The figure shows three views and two pictorial views of one solid part (mm, origin at its lowest corner). Answer the questions. A direction names the side the tool comes from. Give positions to 0.01 mm unless a question says otherwise; leave off trailing zeros. Write each loop counter-clockwise with the first axis right and the second up, starting at its lowest first coordinate (ties: lowest second). Pieces come first, ordered by that corner, then holes. Notation, with made-up numbers: (83.5, 18) - (110.5, 18) arc R23 ccw to (110.5, 35) - close; hole circle Ø4 at (43, 8). An arc over 180 degrees is marked (long way). One line per question, with ' | ' between items. Start each with the question number.
1. A cutting plane is placed at C-C (x = 1.5). Determine the outline of the cut face in (y, z).
2. Given P1, Ø1, axis at x = 1.5, z = 5.5, coming from the -Y side; P2, Ø1, axis at x = 10.5, z = 7, coming from the -Y side; P3, Ø5, axis at x = 11.5, z = 4, coming from the -Y side, each flat-ended and moving along its own axis, determine where each tip first touches the part or whether it passes through.
3. A cutting plane is placed at D-D (x = 10). Determine the outline of the cut face in (y, z), then the cut area to 3 significant figures.
4. Find the intervals of material crossed by L1, parallel to Z at x = 2.25, y = 4.75; L2, parallel to Z at x = 6.75, y = 6.75; L3, parallel to Y at x = 7.75, z = 3, in increasing order. Write a range as from..to.
5. A cutting plane is placed at A-A (y = 4.7). Determine the outline of the cut face in (x, z), then the cut area to 3 significant figures.
6. For the marked faces 1 and 2, determine the directions among +Z, -Z, +X, -X, +Y, -Y from which every point of the face is accessible in a straight line to the end or side of a thin tool.
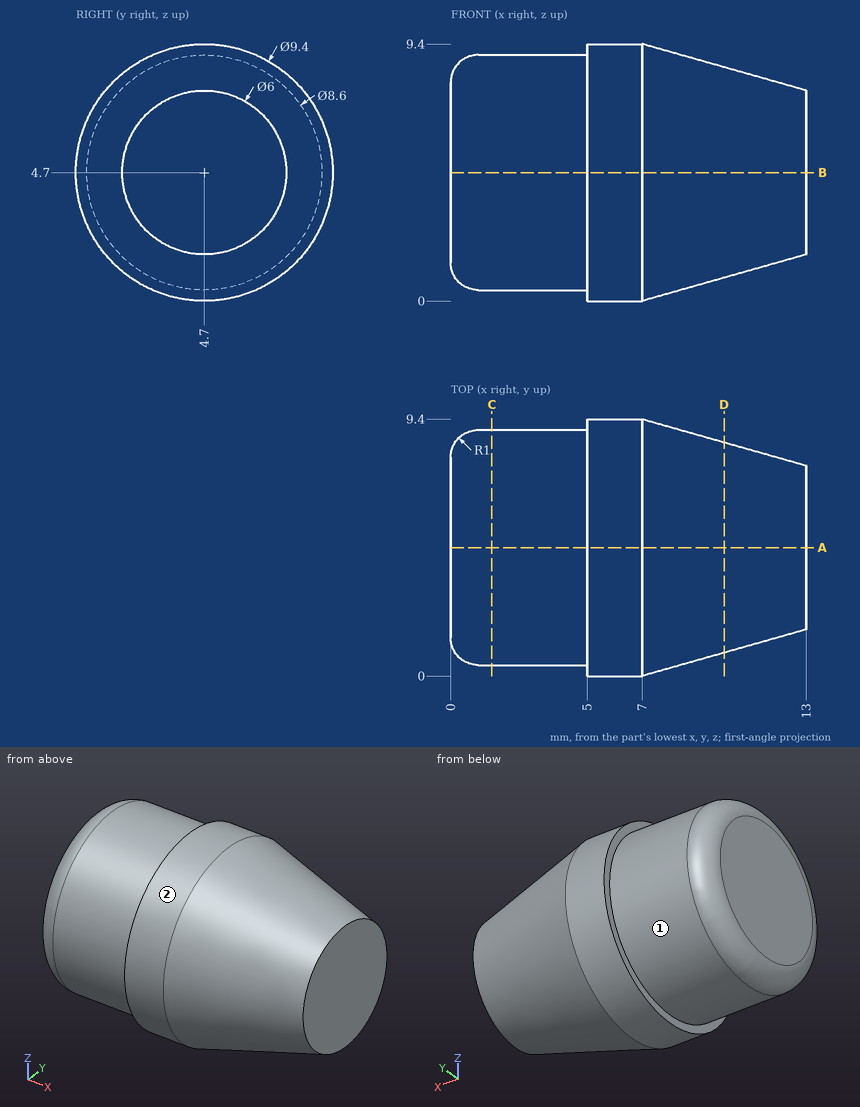
Determined:
1) outline: circle Ø8.6 at (4.7, 4.7)
2) P1: y = 0.41 | P2: y = 1.41 | P3: y = 0.59
3) outline: circle Ø7.7 at (4.7, 4.7) | area: 46.6 mm2
4) L1: 0.4..9 | L2: 0.47..8.93 | L3: 0.55..8.85
5) outline: (0, 1.4) arc R1 ccw to (1, 0.4) - (5, 0.4) - (5, 0) - (7, 0) - (13, 1.7) - (13, 7.7) - (7, 9.4) - (5, 9.4) - (5, 9) - (1, 9) arc R1 ccw to (0, 8) - close | area: 108 mm2
6) face 1: -X | face 2: +X, -X
